```python
from build123d import *

# Parameters (mm, degrees)
EXTRUDE_1_DEPTH = 7.8
SKETCH_4_R      = 2.8
EXTRUDE_3_DEPTH = 4
SKETCH_5_W      = 7
SKETCH_5_H      = 4
EXTRUDE_4_DEPTH = 12
SKETCH_7_W      = 19.6
SKETCH_7_H      = 4.4
EXTRUDE_5_DEPTH = 2
FILLET_2_R      = 1
HOLE_WIZARD_1_D = 1.3
FILLET_3_R      = 1.5


with BuildPart() as part:
    # 草图1 → 凸台-拉伸1 (new, symmetric)
    with BuildSketch(Plane.XY):
        with BuildLine():
            Line((5, 0), (5, 90))
            Line((5, 90), (-5, 90))
            Line((-5, 90), (-5, 0))
            ThreePointArc((-5, 0), (0, -5), (5, 0))
        make_face()
    extrude(amount=EXTRUDE_1_DEPTH, both=True)

    # 草图4 → 凸台-拉伸3 (add)
    with BuildSketch(Plane.XY.offset(7.8)):
        Circle(SKETCH_4_R)
    extrude_3 = extrude(amount=EXTRUDE_3_DEPTH)

    # 草图5 → 凸台-拉伸4 (add)
    with BuildSketch(Plane(origin=(0, 102, 0), x_dir=(1, 0, 0), z_dir=(0, 1, 0))):
        Rectangle(SKETCH_5_W, SKETCH_5_H)
    extrude(amount=-EXTRUDE_4_DEPTH)

    # 草图7 → 凸台-拉伸5 (add, symmetric)
    with BuildSketch(Plane.XY):
        with Locations((0, 99.8)):
            Rectangle(SKETCH_7_W, SKETCH_7_H)
    extrude(amount=EXTRUDE_5_DEPTH, both=True)

    # 草图10 → 切除-旋转1 (revolve, cut)
    with BuildSketch(Plane.XY):
        with BuildLine():
            ThreePointArc((4.15, 102), (2.934493142, 104.934493142), (0, 106.15))
            Line((0, 106.15), (0, 102))
            Line((0, 102), (0, 97.85))
            ThreePointArc((0, 97.85), (2.934493142, 99.065506858), (4.15, 102))
        make_face()
    revolve(axis=Axis((0, 106.15, 0), (0, -1, 0)), mode=Mode.SUBTRACT)

    # 镜向2: 凸台-拉伸3 across plane
    add(extrude_3.mirror(Plane.XY))

    # 圆角2
    fillet_2_edges = [part.edges().sort_by_distance(p)[0] for p in [
        (-9.8, 97.6, 0),
        (9.8, 97.6, 0),
    ]]
    fillet(fillet_2_edges, radius=FILLET_2_R)

    # 孔1 (through all)
    with Locations(Plane(origin=(0, 97.6, 0), x_dir=(-1, 0, 0), z_dir=(0, -1, 0))):
        with Locations((5.65, 0), (-5.65, 0)):
            Hole(HOLE_WIZARD_1_D / 2)

    # 圆角3
    fillet_3_edges = [part.edges().sort_by_distance(p)[0] for p in [
        (0, 90, -2),
        (-3.5, 90, 0),
        (0, 90, 2),
        (3.5, 90, 0),
    ]]
    fillet(fillet_3_edges, radius=FILLET_3_R - 0.0001)  # a hair under: the kernel refuses the full size


solid = part.part
```
Can you work these out from the model? Positions are in its coordinate system, mm. A direction names the side the tool comes from. Give positions to 0.01 mm unless a question says otherwise; leave off trailing zeros. Loops run counter-clockwise (first coordinate to the right, second up) from the corner with the lowest first, then second, coordinate; pieces in that order, holes last. Notation, with made-up numbers: M 32.5,-2.75 L 54.5,-2.75 A27 ccw 54.5,36.25 Z; hole C 16.25,-32.5 d7. An arc over 180 degrees is marked long. Answer in a Markdown table with one row per item.
1. Suppose I cut it at B-B on y = 54.5. Write out the boundary of the cut face in (x, z), plus the area to 3 significant figures.
Taken from the geometry:
| item | result |
|---|---|
| outline | M -5,-7.8 L 5,-7.8 L 5,7.8 L -5,7.8 Z |
| area | 156 mm² |
2. Suppose I cut it at C-C on z = -5.5. Write out the boundary of the cut face in (x, y), plus the area to 3 significant figures.
Taken from the geometry:
| item | result |
|---|---|
| outline | M -5,0 A5 ccw 5,0 L 5,90 L -5,90 Z |
| area | 939 mm² |
3. For pin 1 Ø2 at (y, z) = (95.5, 1) entering from +X; pin 2 Ø8 at (x, z) = (-7, -6.5) entering from -Y; pin 3 Ø12 at (y, z) = (87, -2.5) entering from -X, each with a flat end and sliding along its axis, tell me the tip position at first contact or that it passes through.
Taken from the geometry:
| item | result |
|---|---|
| pin 1 | stops at x = 3.5 |
| pin 2 | stops at y = -4 |
| pin 3 | stops at x = -5 |
4. If I drill on line 1 along Z through (x, y) = (-5.65, 100.95); line 2 along Y through (x, z) = (-8, 0); line 3 along Z through (x, y) = (-3, 26), over which ranges is the centre line in solid material (lowest first)?
Taken from the geometry:
| item | result |
|---|---|
| line 1 | z = -2 to -0.65, 0.65 to 2 |
| line 2 | y = 97.6 to 102 |
| line 3 | z = -7.8 to 7.8 |
5. Suppose I cut it at A-A on x = 0. Write out the boundary of the cut face in (y, z), plus the area to 3 significant figures.
Taken from the geometry:
| item | result |
|---|---|
| outline | M -5,-7.8 L -2.8,-7.8 L -2.8,-11.8 L 2.8,-11.8 L 2.8,-7.8 L 90,-7.8 L 90,-3.5 A1.5 cw 91.5,-2 L 98.36,-2 A4.15 cw 98.36,2 L 91.5,2 A1.5 cw 90,3.5 L 90,7.8 L 2.8,7.8 L 2.8,11.8 L -2.8,11.8 L -2.8,7.8 L -5,7.8 Z |
| area | 1,560 mm² |
6. Which directions (+Z, -Z, +X, -X, +Y, -Y) give clear straight access to the entire face, cutting with the end or side of a thin tool? Please do faces 5 (the flat face through (5, 44, 0)), 6 (the flat face through (0, 98, -2)), 7 (the flat face through (0, 98, 2)), 8 (the flat face through (-5, 46, 0)), 9 (the flat face through (3.5, 95, 0)).
Taken from the geometry:
| item | result |
|---|---|
| face 5 | +Z, -Z, +X, -Y |
| face 6 | -Z, +X, -X, +Y |
| face 7 | +Z, +X, -X, +Y |
| face 8 | +Z, -Z, -X, -Y |
| face 9 | +Z, -Z, +X |
7. Thinking about a two-plate mould opening in Y: for faces 1 (the flat face through (-3.5, 95, 0)), 2 (the cylindrical face through (0, -5, 0)), 3 (the flat face through (-7, 97.6, 0)), 4 (the cylindrical face through (-2.8, 0.1, 9.8)), which applies, released by +Y, released by -Y, zero draft, split by the parting line, or undercut?
Taken from the geometry:
| item | result |
|---|---|
| face 1 | undercut |
| face 2 | released by -Y |
| face 3 | undercut |
| face 4 | split by the parting line |
